Here's how the part is built. I have some questions about the finished solid (model axes, mm). Face numbers are marked on the shaded views. A direction names the side the tool comes from. Round coordinates to 2 decimals unless told otherwise and drop trailing zeros. Order: outer loops, then holes, each group sorted by start corner. A loop starts at its lowest first (then second) coordinate and runs counter-clockwise, first axis right, second up. Notation, with made-up numbers: (19, -16.75) -> (50, -16.75) arc R29 cw to (50, 21.25) -> close; hole circle Ø9 at (29.5, -29). An arc over 180 degrees is marked (long way). Answer in a Markdown table with one row per item.
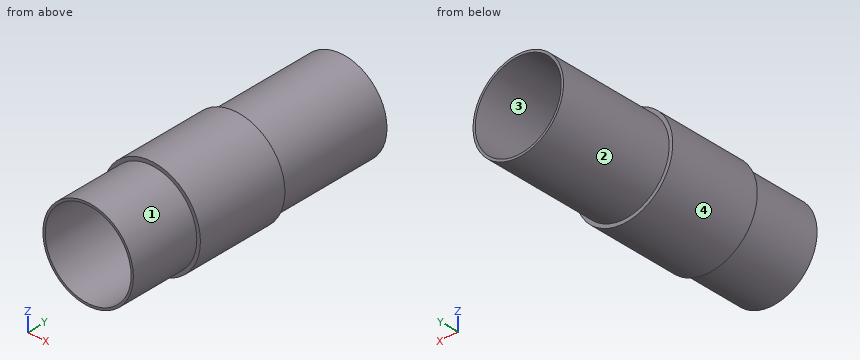
```python
from build123d import *

# Parameters (mm, degrees)
SKETCH1_R           = 25.0063
SKETCH1_R_2         = 23.749
BOSS_EXTRUDE1_DEPTH = 152.4
SKETCH5_R           = 27.0002
SKETCH5_R_2         = 25.0063
BOSS_EXTRUDE3_DEPTH = 50.8


with BuildPart() as part:
    # Sketch1 → Boss-Extrude1 (new body)
    with BuildSketch(Plane(origin=(0, 0, 0), x_dir=(1, 0, 0), z_dir=(0, 1, 0))):
        Circle(SKETCH1_R)
        Circle(SKETCH1_R_2, mode=Mode.SUBTRACT)
    extrude(amount=BOSS_EXTRUDE1_DEPTH)

    # Sketch5 → Boss-Extrude3 (add)
    with BuildSketch(Plane(origin=(0, 88.9, 0), x_dir=(1, 0, 0), z_dir=(0, 1, 0))):
        Circle(SKETCH5_R)
        Circle(SKETCH5_R_2, mode=Mode.SUBTRACT)
    extrude(amount=-BOSS_EXTRUDE3_DEPTH)


solid = part.part
```
1. For the marked faces 1 and 2, which set-ups out of +Z, -Z, +X, -X, +Y, -Y let a thin tool reach every point of the face, with its end or its side?
Numbers:
| item | result |
|---|---|
| face 1 | -Y |
| face 2 | +Y |
2. Suppose I cut it at B-B on x = 0. Write out the boundary of the cut face in (y, z), then the cut area to 3 significant figures.
Numbers:
| item | result |
|---|---|
| outline | (0, -25.01) -> (38.1, -25.01) -> (38.1, -27) -> (88.9, -27) -> (88.9, -25.01) -> (152.4, -25.01) -> (152.4, -23.75) -> (0, -23.75) -> close; (0, 23.75) -> (152.4, 23.75) -> (152.4, 25.01) -> (88.9, 25.01) -> (88.9, 27) -> (38.1, 27) -> (38.1, 25.01) -> (0, 25.01) -> close |
| area | 586 mm2 |
3. Please list where these lines run through material, in increasing order: line 1 along Z through (x, y) = (1, 61.5); line 2 along Z through (x, y) = (0, 94).
Numbers:
| item | result |
|---|---|
| line 1 | z = -26.98 to -23.73, 23.73 to 26.98 |
| line 2 | z = -25.01 to -23.75, 23.75 to 25.01 |
4. Suppose I cut it at C-C on y = 42. Write out the boundary of the cut face in (x, z), then the cut area to 3 significant figures.
Numbers:
| item | result |
|---|---|
| outline | circle Ø54 at (0, 0); hole circle Ø47.5 at (0, 0) |
| area | 518 mm2 |
5. For pin 1 Ø6 at (y, z) = (95.5, -11.5) entering from +X; pin 2 Ø5 at (y, z) = (52, 14) entering from +X; pin 3 Ø12 at (x, y) = (-6.5, 48.5) entering from -Z, each with a flat end and sliding along its axis, tell me the tip position at first contact or that it passes through.
Numbers:
| item | result |
|---|---|
| pin 1 | stops at x = 23.52 |
| pin 2 | stops at x = 24.43 |
| pin 3 | stops at z = -27 |
6. We'd pull the mould along Z, two halves only. Please class the marked faces 3 and 4: released by +Z, released by -Z, zero draft, split by the parting line, or undercut.
Numbers:
| item | result |
|---|---|
| face 3 | undercut |
| face 4 | split by the parting line |
7. Suppose I cut it at A-A on z = 0. Write out the boundary of the cut face in (x, y), then the cut area to 3 significant figures.
Numbers:
| item | result |
|---|---|
| outline | (-27, 38.1) -> (-25.01, 38.1) -> (-25.01, 0) -> (-23.75, 0) -> (-23.75, 152.4) -> (-25.01, 152.4) -> (-25.01, 88.9) -> (-27, 88.9) -> close; (23.75, 0) -> (25.01, 0) -> (25.01, 38.1) -> (27, 38.1) -> (27, 88.9) -> (25.01, 88.9) -> (25.01, 152.4) -> (23.75, 152.4) -> close |
| area | 586 mm2 |
